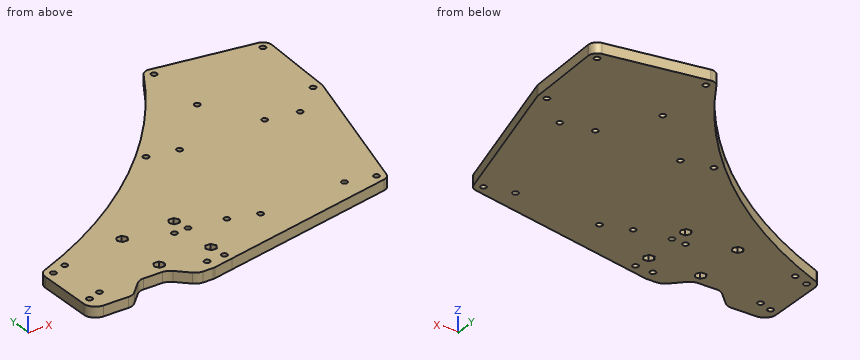
from build123d import *

# Parameters (mm, degrees)
SKETCH2_R           = 2.499965
SKETCH2_R_2         = 2.49997
SKETCH2_R_3         = 2.4999655
SKETCH2_R_4         = 2.499962807
SKETCH2_R_5         = 2.4999705
SKETCH2_R_6         = 2.499967809
SKETCH2_R_7         = 2.499966
SKETCH2_R_8         = 2.4999665
SKETCH2_R_9         = 2.499966488
BOSS_EXTRUDE1_DEPTH = 9
CUT_EXTRUDE1_DEPTH  = 10
CUT_EXTRUDE2_DEPTH  = 244.998875453
SKETCH5_R           = 2.5
CUT_EXTRUDE3_DEPTH  = 244.998875453
CUT_EXTRUDE5_DEPTH  = 10
FILLET1_R           = 10
CUT_EXTRUDE7_DEPTH  = 244.998875453


with BuildPart() as part:
    # Sketch2 → Boss-Extrude1 (new body)
    with BuildSketch(Plane.XY):
        Polygon((-211.70586, -139.55845), (122.983766, -139.55845), (211.70583, 139.558464), (-211.70586, 139.558464), align=None)
        with Locations((-192.444718, -125.900476)):
            Circle(SKETCH2_R, mode=Mode.SUBTRACT)
        with Locations((-181.028235, -121.988219)):
            Circle(SKETCH2_R_2, mode=Mode.SUBTRACT)
        with Locations((-192.0409685, -80.3042345)):
            Circle(SKETCH2_R_3, mode=Mode.SUBTRACT)
        with Locations((-179.0281635, -75.623296193)):
            Circle(SKETCH2_R_4, mode=Mode.SUBTRACT)
        with Locations((-92.3000565, -128.9494755)):
            Circle(SKETCH2_R_5, mode=Mode.SUBTRACT)
        with Locations((-76.832143809, -128.336904809)):
            Circle(SKETCH2_R_6, mode=Mode.SUBTRACT)
        with Locations((-87.928392809, -81.863553809)):
            Circle(SKETCH2_R_6, mode=Mode.SUBTRACT)
        with Locations((-75.718345809, -81.250965809)):
            Circle(SKETCH2_R_6, mode=Mode.SUBTRACT)
        with Locations((-45.325502, -86.123854)):
            Circle(SKETCH2_R, mode=Mode.SUBTRACT)
        with Locations((-21.323083, -93.781229)):
            Circle(SKETCH2_R_7, mode=Mode.SUBTRACT)
        with Locations((54.304011, -89.994307)):
            Circle(SKETCH2_R_7, mode=Mode.SUBTRACT)
        with Locations((78.1115035, -95.7303835)):
            Circle(SKETCH2_R_8, mode=Mode.SUBTRACT)
        with Locations((114.776659, 36.09363)):
            Circle(SKETCH2_R, mode=Mode.SUBTRACT)
        with Locations((86.96623, 12.266557)):
            Circle(SKETCH2_R_7, mode=Mode.SUBTRACT)
        with Locations((59.4275, 17.097677)):
            Circle(SKETCH2_R, mode=Mode.SUBTRACT)
        with Locations((-40.842451, 21.163049)):
            Circle(SKETCH2_R, mode=Mode.SUBTRACT)
        with Locations((-15.2807135, 15.9838705)):
            Circle(SKETCH2_R_8, mode=Mode.SUBTRACT)
        with Locations((32.626661, 62.749598)):
            Circle(SKETCH2_R_7, mode=Mode.SUBTRACT)
        with Locations((118.780878488, 104.469667)):
            Circle(SKETCH2_R_9, mode=Mode.SUBTRACT)
        with Locations((32.7798015, 116.8664005)):
            Circle(SKETCH2_R_8, mode=Mode.SUBTRACT)
    extrude(amount=BOSS_EXTRUDE1_DEPTH)

    # Sketch3 → Cut-Extrude1 (cut)
    with BuildSketch(Plane.XY.offset(9)):
        Polygon((147.113293383, 124.3664005), (73.705987484, -139.55845), (211.70583, -139.55845), (211.70583, 139.558464), (-211.70586, 139.558464), (-211.70586, -139.55845), (-199.944718, -139.55845), (-199.944718, -77.260214262), (29.956914073, 124.3664005), align=None)
    extrude(amount=-CUT_EXTRUDE1_DEPTH, mode=Mode.SUBTRACT)

    # Sketch4 → Cut-Extrude2 (cut, through all)
    with BuildSketch(Plane.XY.offset(9)):
        Polygon((-163.885127, -139.55845), (-147.880898, -123.554221), (-123.333708966, -123.554221), (-107.329479966, -139.55845), align=None)
    extrude(amount=-CUT_EXTRUDE2_DEPTH, mode=Mode.SUBTRACT)

    # Sketch5 → Cut-Extrude3 (cut, through all)
    with BuildSketch(Plane.XY.offset(9)):
        with Locations((-123.130898, -113.554221)):
            Circle(SKETCH5_R)
        with Locations((-78.130898, -113.554221)):
            Circle(SKETCH5_R)
        with Locations((-123.380898, -67.554221)):
            Circle(SKETCH5_R)
        with Locations((-78.130898, -67.554221)):
            Circle(SKETCH5_R)
    extrude(amount=-CUT_EXTRUDE3_DEPTH, mode=Mode.SUBTRACT)

    # Sketch6 → Cut-Extrude5 (cut)
    with BuildSketch(Plane.XY.offset(9)):
        with BuildLine():
            Line((-195.525508542, -73.384512142), (-194.933621691, -73.384512142))
            ThreePointArc((-194.933621691, -73.384512142), (-115.656074248, -30.741284252), (-46.149790694, 26.462307945))
            ThreePointArc((-46.149790694, 26.462307945), (-6.887258575, 71.211725192), (26.296691523, 120.637247226))
            Line((26.296691523, 120.637247226), (26.296691523, 121.156339417))
            Line((26.296691523, 121.156339417), (-195.525508542, -73.384512142))
        make_face()
        Polygon((147.113293383, 35.655168177), (147.113293383, 124.3664005), (122.439403996, 35.655168177), align=None)
        Polygon((-75.287663516, -135.676154132), (-93.736030822, -139.55845), (73.705987484, -139.55845), (83.854883116, -103.069632849), (79.655983667, -103.069632849), align=None)
        with BuildLine():
            Line((79.655983667, -103.069632849), (83.854883116, -103.069632849))
            Line((83.854883116, -103.069632849), (85.337218021, -97.740122205))
            ThreePointArc((85.337218021, -97.740122205), (83.24278011, -101.200301265), (79.655983667, -103.069632849))
        make_face()
        with BuildLine():
            ThreePointArc((-196.986177186, -74.665536862), (-196.011897332, -73.941709513), (-194.933621691, -73.384512142))
            Line((-194.933621691, -73.384512142), (-195.525508542, -73.384512142))
            Line((-195.525508542, -73.384512142), (-196.986177186, -74.665536862))
        make_face()
        Polygon((26.296691523, 124.3664005), (26.296691523, 121.156339417), (27.834592626, 122.505097973), (29.956914073, 124.3664005), align=None)
        with BuildLine():
            Line((27.834592626, 122.505097973), (26.296691523, 121.156339417))
            Line((26.296691523, 121.156339417), (26.296691523, 120.637247226))
            ThreePointArc((26.296691523, 120.637247226), (26.989824424, 121.633597313), (27.834592626, 122.505097973))
        make_face()
        with BuildLine():
            Line((29.956914073, 124.3664005), (27.834592626, 122.505097973))
            ThreePointArc((27.834592626, 122.505097973), (30.137854408, 123.885667952), (32.779801516, 124.3664005))
            Line((32.779801516, 124.3664005), (29.956914073, 124.3664005))
        make_face()
        with BuildLine():
            Line((147.113293383, 124.3664005), (32.779801516, 124.3664005))
            ThreePointArc((32.779801516, 124.3664005), (33.31619378, 124.347194798), (33.849838899, 124.289676055))
            Line((33.849838899, 124.289676055), (119.850915887, 111.892942555))
            ThreePointArc((119.850915887, 111.892942555), (124.449885477, 109.380100764), (126.280878488, 104.469667))
            ThreePointArc((126.280878488, 104.469667), (126.277670913, 104.250342289), (126.268050933, 104.031205177))
            Line((126.268050933, 104.031205177), (122.263831446, 35.655168177))
            Line((122.263831446, 35.655168177), (122.439403996, 35.655168177))
            Line((122.439403996, 35.655168177), (147.113293383, 124.3664005))
        make_face()
        with BuildLine():
            Line((122.002373456, 34.083891063), (122.439403996, 35.655168177))
            Line((122.439403996, 35.655168177), (122.263831446, 35.655168177))
            ThreePointArc((122.263831446, 35.655168177), (122.174935028, 34.862568747), (122.002373456, 34.083891063))
        make_face()
    extrude(amount=-CUT_EXTRUDE5_DEPTH, mode=Mode.SUBTRACT)

    # Fillet1
    # the kernel refuses this fillet: 10 mm, written as the material it adds along each edge
    with BuildSketch(Plane(origin=(-147.880898, -123.554221, 9), x_dir=(1, 0, 0), z_dir=(0, 0, -1)), Plane(origin=(-123.333708966, -123.554221, 9), x_dir=(0.707106781186551, -0.7071067811865441, 0), z_dir=(0, 0, -1))) as fillet1_piece_1:
        with BuildLine():
            CenterArc((FILLET1_R * 0.414213562373, FILLET1_R), FILLET1_R, 225, 45)
            Line((-FILLET1_R * 0.292893218813, FILLET1_R * 0.292893218813), (0, 0))
            Line((0, 0), (FILLET1_R * 0.414213562373, 0))
        make_face()
    extrude(amount=9)
    # the kernel refuses this fillet: 10 mm, written as the material it takes off along each edge
    with BuildSketch(Plane(origin=(-199.944718, -77.260214262, 20.264688934), x_dir=(0, -1, 0), z_dir=(0, 0, -1))) as fillet1_2_piece_1:
        with BuildLine():
            CenterArc((4.505875574, -10), FILLET1_R, 90, 45.239414653)
            Line((-2.5946774, -2.958540814), (0, 0))
            Line((0, 0), (4.505875574, 0))
        make_face()
    extrude(amount=31.529377868, mode=Mode.SUBTRACT)
    with BuildSketch(Plane(origin=(-163.885127, -139.55845, 19.355339059), x_dir=(-1, 0, 0), z_dir=(0, 0, -1)), Plane(origin=(-107.329479966, -139.55845, 19.355339059), x_dir=(-0.707106781186551, 0.7071067811865441, 0), z_dir=(0, 0, -1))) as fillet1_2_piece_2:
        with BuildLine():
            CenterArc((FILLET1_R * 0.414213562373, FILLET1_R), FILLET1_R, 225, 45)
            Line((-FILLET1_R * 0.292893218813, FILLET1_R * 0.292893218813), (0, 0))
            Line((0, 0), (FILLET1_R * 0.414213562373, 0))
        make_face()
    extrude(amount=29.710678119, mode=Mode.SUBTRACT)
    with BuildSketch(Plane(origin=(-93.736030822, -139.55845, 11.602018692), x_dir=(-1, 0, 0), z_dir=(0, 0, -1))) as fillet1_2_piece_3:
        with BuildLine():
            CenterArc((FILLET1_R * 0.104080747675, FILLET1_R), FILLET1_R, 258.116013885, 11.883986115)
            Line((-FILLET1_R * 0.101849941288, FILLET1_R * 0.0214334200765), (0, 0))
            Line((0, 0), (FILLET1_R * 0.104080747675, 0))
        make_face()
    extrude(amount=14.204037384, mode=Mode.SUBTRACT)
    with BuildSketch(Plane(origin=(-199.944718, -139.55845, 34), x_dir=(1, 0, 0), z_dir=(0, 0, -1))) as fillet1_2_piece_4:
        with BuildLine():
            CenterArc((FILLET1_R, -FILLET1_R), FILLET1_R, 90, 90)
            Line((0, -FILLET1_R), (0, 0))
            Line((0, 0), (FILLET1_R, 0))
        make_face()
    extrude(amount=59, mode=Mode.SUBTRACT)

    # Sketch7 → Cut-Extrude7 (cut, through all)
    with BuildSketch(Plane.XY):
        Polygon((-118.512095846, -113.554221), (-120.821496923, -109.554221), (-125.440299077, -109.554221), (-127.749700154, -113.554221), (-125.440299077, -117.554221), (-120.821496923, -117.554221), align=None)
        Polygon((-82.749700154, -113.554221), (-80.440299077, -117.554221), (-75.821496923, -117.554221), (-73.512095846, -113.554221), (-75.821496923, -109.554221), (-80.440299077, -109.554221), align=None)
        Polygon((-80.440299077, -71.554221), (-75.821496923, -71.554221), (-73.512095846, -67.554221), (-75.821496923, -63.554221), (-80.440299077, -63.554221), (-82.749700154, -67.554221), align=None)
        Polygon((-121.071496923, -71.554221), (-118.762095846, -67.554221), (-121.071496923, -63.554221), (-125.690299077, -63.554221), (-127.999700154, -67.554221), (-125.690299077, -71.554221), align=None)
    extrude(amount=CUT_EXTRUDE7_DEPTH, mode=Mode.SUBTRACT)


solid = part.part
Could you check a few things on this model? Use its own coordinates, in mm. Round coordinates to 2 decimals unless told otherwise and drop trailing zeros. Order: outer loops, then holes, each group sorted by start corner. A loop starts at its lowest first (then second) coordinate and runs counter-clockwise, first axis right, second up.
Q1. Please list where these lines run through material, in increasing order: probe 1 along Y at (x, z) = (-75, 4.75); probe 2 along Y at (x, z) = (52.5, 7.25); probe 3 along Y at (x, z) = (-179, 4.25).
Geometry says:
probe 1: y = -135.62 to -130.04, -126.64 to -116.13, -110.98 to -83.65, -78.86 to -70.13, -64.98 to -0.08
probe 2: y = -108.78 to -91.73, -88.26 to 121.6
probe 3: y = -139.56 to -123.45, -120.53 to -78.12, -73.12 to -66.37
Q2. Imagine slicing it at A-A, the plane y = -42.5. List the corners of the cut face in (x, z) for me.
Geometry says:
outline: (-134.11, 0) - (100.7, 0) - (100.7, 9) - (-134.11, 9) - close
Q3. Imagine slicing it at C-C, the plane z = 5.25. State how many separate pieces and enclosed holes the cut face has, then the cut area to 3 significant figures.
Geometry says:
separate pieces: 1
enclosed holes: 24
area: 47,900 mm2
Q4. Imagine slicing it at B-B, the plane x = -53.5. List the corners of the cut face in (y, z) for me, then the cut area to 3 significant figures.
Geometry says:
outline: (-131.09, 0) - (19.26, 0) - (19.26, 9) - (-131.09, 9) - close
area: 1,350 mm2
Q5. I'm going to push flat-ended pins straight in: P1, Ø2, axis at x = 31.5, z = 4, coming from the -Y side; P2, Ø2.5, axis at x = -124.5, z = 2.5, coming from the +Y side; P3, Ø1.4, axis at x = -123, z = 5, coming from the -Y side. Where does each tip first touch, or does it pass through?
Geometry says:
P1: stops at y = -113.41
P2: stops at y = -35.73
P3: stops at y = -125
